Read the model definition and answer for the solid it produces. Units are mm, in the model's axes. A direction names the side the tool comes from. Give positions to 0.01 mm unless a question says otherwise; leave off trailing zeros. Order: outer loops, then holes, each group sorted by start corner. A loop starts at its lowest first (then second) coordinate and runs counter-clockwise, first axis right, second up. Notation, with made-up numbers: (16, 14.25) - (58, 14.25) arc R4 ccw to (58, 21.25) - close; hole circle Ø11 at (58, 45.25). An arc over 180 degrees is marked (long way). Return JSON: item names as keys, results as strings.
```python
from build123d import *

# Parameters (mm, degrees)
F0_W            = 790
F0_H            = 6
F2_W            = 790
F2_H            = 8
F5_D            = 22
F5_COPIES_COUNT = 16


# Not quite as in the source:
# - a pattern or mirror of a feature is missing from the dataset's text; its kind, count and spacing are read off the source's solid


with BuildPart() as f1:
    # F0 (on Front) → F1 (revolve)
    with BuildSketch(Plane.XZ):
        Polygon((-450, 490), (-450, 420), (450, 420), (450, 445), (-410, 445), (-410, 490), align=None)
        with Locations((-15, 435)):
            Rectangle(F0_W, F0_H, mode=Mode.SUBTRACT)
    revolve(axis=Axis((-71.5964585543, 0, 0), (1, 0, 0)))

    # F2 (on Front) → F3 (revolve, cut)
    with BuildSketch(Plane.XZ):
        with Locations((-15, 434)):
            Rectangle(F2_W, F2_H)
    revolve(axis=Axis((-160.7926189899, 0, 0), (1, 0, 0)), mode=Mode.SUBTRACT)

    # F5 (through all)
    with Locations(Plane(origin=(-450, 0, 0), x_dir=(0, -1, 0), z_dir=(-1, 0, 0))):
        with Locations((-232.5, 402.7018127598)):
            f5 = Hole(F5_D / 2)

    # F5_copies: F5 ×16 about axis
    f5_copies_axis = Axis((0, 0, 0), (1, 0, 0))
    for i in range(1, F5_COPIES_COUNT):
        add(f5.rotate(f5_copies_axis, i * 360 / F5_COPIES_COUNT), mode=Mode.SUBTRACT)


solid = f1.part
```
Q1. A cutting plane is placed at A-A (z = 0). Write down the section's boundary in (x, y), and give its area (3 significant figures).
Values:
{"outline": "(-450, -490) - (-410, -490) - (-410, -445) - (450, -445) - (450, -420) - (-450, -420) - close; (-450, 420) - (450, 420) - (450, 445) - (-410, 445) - (-410, 490) - (-450, 490) - close; hole (-410, -438) - (380, -438) - (380, -430) - (-410, -430) - close; hole (-410, 430) - (380, 430) - (380, 438) - (-410, 438) - close", "area": "36,000 mm²"}
Q2. Determine the mould class of faces 1 (the cylindrical face through (6.3, -126.157, 400.605)), 2 (the flat face through (-450, 361, 215)), 3 (the cylindrical face through (-430.28, 478.35, -106.22)) for opening direction Z: released by +Z, released by -Z, zero draft, split by the parting line, or undercut.
Values:
{"face 1": "undercut", "face 2": "zero draft", "face 3": "split by the parting line"}
Q3. A cutting plane is placed at C-C (x = 296). Write down the section's boundary in (y, z), and give its area (3 significant figures).
Values:
{"outline": "circle Ø890 at (0, 0); circle Ø860 at (0, 0); hole circle Ø876 at (0, 0); hole circle Ø840 at (0, 0)", "area": "46,100 mm²"}
Q4. Given pin 1 (17.5 mm diameter, centred on y = 402.7, z = -232.5, fed in from -X); pin 2 (2 mm diameter, centred on x = -230, y = -311.5, fed in from +Z); pin 3 (12 mm diameter, centred on x = -189.5, z = -357.5, fed in from -Y); pin 4 (1.5 mm diameter, centred on x = 277.5, z = 190.5, fed in from +Y), each flat-ended and moving along its own axis, determine where each tip first touches the part or whether it passes through.
Values:
{"pin 1": "passes through", "pin 2": "stops at z = 318.77", "pin 3": "stops at y = -272.9", "pin 4": "stops at y = 402.52"}
Q5. Consider L1, parallel to Y at x = -146, z = 0; L2, parallel to X at y = 339, z = 274.5. Determine where each line is inside the solid, lowest interval first.
Values:
{"L1": "y = -445 to -438, -430 to -420, 420 to 430, 438 to 445", "L2": "x = -450 to -410, 380 to 450"}
Q6. For faces 4 (the cylindrical face through (13.98, -441.213, -57.93)), 5 (the flat face through (380, 322, -290)), 6 (the flat face through (450, -266, -328)), determine the directions among +Z, -Z, +X, -X, +Y, -Y from which every point of the face is accessible in a straight line to the end or side of a thin tool.
Values:
{"face 4": "+X", "face 5": "none", "face 6": "+Z, -Z, +X, +Y, -Y"}
